```python
from build123d import *

# Parameters (mm, degrees)
F1_DEPTH = 125


with BuildPart() as f1:
    # F0 (on Front) → F1 (new body, symmetric)
    with BuildSketch(Plane.XZ):
        with BuildLine():
            Line((0, 100), (0, 0))
            Line((0, 0), (7.5, 0))
            Line((7.5, 0), (7.5, 75.160644))
            ThreePointArc((7.5, 75.160644), (10.652672, 83.267727), (18.454131, 87.114981))
            Line((18.454131, 87.114981), (40, 89))
            Line((40, 89), (40, 100))
            Line((40, 100), (0, 100))
        make_face()
        with BuildLine():
            Line((80, 100), (40, 100))
            Line((40, 100), (40, 89))
            Line((40, 89), (74.522934, 92.020365))
            ThreePointArc((74.522934, 92.020365), (78.423664, 93.943992), (80, 97.997534))
            Line((80, 97.997534), (80, 100))
        make_face()
        with BuildLine():
            Line((7.5, 0), (0, 0))
            Line((0, 0), (0, -100))
            Line((0, -100), (40, -100))
            Line((40, -100), (40, -89))
            Line((40, -89), (18.454131, -87.114981))
            ThreePointArc((18.454131, -87.114981), (10.652672, -83.267727), (7.5, -75.160644))
            Line((7.5, -75.160644), (7.5, 0))
        make_face()
        with BuildLine():
            Line((40, -89), (40, -100))
            Line((40, -100), (80, -100))
            Line((80, -100), (80, -97.997534))
            ThreePointArc((80, -97.997534), (78.423664, -93.943992), (74.522934, -92.020365))
            Line((74.522934, -92.020365), (40, -89))
        make_face()
    extrude(amount=F1_DEPTH, both=True)


solid = f1.part
```
Model file for the job. Use its own axes, mm. A direction names the side the tool comes from. Give positions to 0.01 mm unless a question says otherwise; leave off trailing zeros. Loops run counter-clockwise (first coordinate to the right, second up) from the corner with the lowest first, then second, coordinate; pieces in that order, holes last. Notation, with made-up numbers: (-25.5, 86.5) -> (25.5, 86.5) arc R8 cw to (25.5, 99.5) -> close; hole circle Ø6 at (-39.5, 26). An arc over 180 degrees is marked (long way). Use CSV: the item, a comma, the result in double quotes. Start each with the question number.
1) Slice it at B-B on y = 63. Give the cut face in (x, z), plus the area to 3 significant figures.
2) Slice it at C-C on z = 54.5. Give the cut face in (x, y), plus the area to 4 significant figures.
3) Wall check: line 1 (X direction, y = 56.5, z = -9.5); line 2 (Z direction, x = 10.5, y = -71.5); line 3 (Z direction, x = 53.5, y = 39). Give the ranges that are in metal, low to high.
4) Slice it at A-A on x = 35. Give the cut face in (y, z), plus the area to 3 significant figures.
5) Flat gauge pin, fed straight in: pin 1 Ø4 at (y, z) = (-21.5, 5) entering from +X. Where does the tip first touch, or does it go through?
6) Tool access for faces 1 (the cylindrical face through (10.569, -1.75, 83.175)), 2 (the flat face through (0, -2, 1)): list every direction of +Z, -Z, +X, -X, +Y, -Y with a clear straight run to the whole face (end or side of a thin tool).
7) Mould opens along Z. For faces 3 (the flat face through (39, -2, -100)), 4 (the flat face through (41, -2, 100)), 5 (the flat face through (7, 125, 8)), 6 (the cylindrical face through (78.466, -1.75, -93.99)) say: released by +Z, released by -Z, zero draft, split by the parting line, or undercut.
8) Slice it at D-D on x = 47.5. Give the cut face in (y, z), plus the area to 3 significant figures.
Computed values:
1,outline,"(0, -100) -> (80, -100) -> (80, -98) arc R6 ccw to (74.52, -92.02) -> (18.45, -87.11) arc R12 cw to (7.5, -75.16) -> (7.5, 75.16) arc R12 cw to (18.45, 87.11) -> (74.52, 92.02) arc R6 ccw to (80, 98) -> (80, 100) -> (0, 100) -> close"
1,area,"3,090 mm^2"
2,outline,"(0, -125) -> (7.5, -125) -> (7.5, 125) -> (0, 125) -> close"
2,area,"1,875 mm^2"
3,line 1,"x = 0 to 7.5"
3,line 2,"z = -100 to -83.1, 83.1 to 100"
3,line 3,"z = -100 to -90.18, 90.18 to 100"
4,outline,"(-125, -100) -> (125, -100) -> (125, -88.56) -> (-125, -88.56) -> close; (-125, 88.56) -> (125, 88.56) -> (125, 100) -> (-125, 100) -> close"
4,area,"5,720 mm^2"
5,pin 1,"stops at x = 7.5"
6,face 1,"+X, +Y, -Y"
6,face 2,"+Z, -Z, -X, +Y, -Y"
7,face 3,"released by -Z"
7,face 4,"released by +Z"
7,face 5,"zero draft"
7,face 6,"undercut"
8,outline,"(-125, -100) -> (125, -100) -> (125, -89.66) -> (-125, -89.66) -> close; (-125, 89.66) -> (125, 89.66) -> (125, 100) -> (-125, 100) -> close"
8,area,"5,170 mm^2"
